Check sheet for the modelled part. Datum: model origin and axes. Units: mm. A direction names the side the tool comes from. Give positions to 0.01 mm unless a question says otherwise; leave off trailing zeros. Order: outer loops, then holes, each group sorted by start corner. A loop starts at its lowest first (then second) coordinate and runs counter-clockwise, first axis right, second up.
```python
from build123d import *

# Parameters (mm, degrees)
ESQUISSE1_W             = 150
ESQUISSE1_H             = 150
BOSS_EXTRU_1_DEPTH      = 5
ESQUISSE2_W             = 12
ESQUISSE2_H             = 60
ESQUISSE2_H_2           = 35
ENL_V_MAT_EXTRU_1_DEPTH = 5


with BuildPart() as part:
    # Esquisse1 → Boss.-Extru.1 (new body)
    with BuildSketch(Plane.XY):
        with Locations((75, 75)):
            Rectangle(ESQUISSE1_W, ESQUISSE1_H)
    extrude(amount=BOSS_EXTRU_1_DEPTH)

    # Esquisse2 → Enlèv. mat.-Extru.1 (cut)
    with BuildSketch(Plane.XY.offset(5)):
        with Locations((26, 90)):
            Rectangle(ESQUISSE2_W, ESQUISSE2_H)
        with Locations((124, 90)):
            Rectangle(ESQUISSE2_W, ESQUISSE2_H)
        with Locations((54, 22.5)):
            Rectangle(ESQUISSE2_W, ESQUISSE2_H_2)
        with Locations((96, 22.5)):
            Rectangle(ESQUISSE2_W, ESQUISSE2_H_2)
    extrude(amount=-ENL_V_MAT_EXTRU_1_DEPTH, mode=Mode.SUBTRACT)


solid = part.part
```
(1) Cross-section at B-B on z = 2.5. Enter the section's corners in (x, y), then the cut area to 3 significant figures.
Response values:
outline: (0, 0) - (150, 0) - (150, 150) - (0, 150) - close; hole (20, 60) - (32, 60) - (32, 120) - (20, 120) - close; hole (48, 5) - (60, 5) - (60, 40) - (48, 40) - close; hole (90, 5) - (102, 5) - (102, 40) - (90, 40) - close; hole (118, 60) - (130, 60) - (130, 120) - (118, 120) - close
area: 20,200 mm2
(2) Cross-section at A-A on y = 87. Enter the section's corners in (x, z).
Response values:
outline: (0, 0) - (20, 0) - (20, 5) - (0, 5) - close; (32, 0) - (118, 0) - (118, 5) - (32, 5) - close; (130, 0) - (150, 0) - (150, 5) - (130, 5) - close
(3) Release check for a two-part mould opening along Y. For faces 1 (the face through (96, 40, 3)), 2 (the face through (74, 150, 2)), 3 (the face through (74, 76, 5)), 4 (the face through (26, 120, 3)) record: released by +Y, released by -Y, zero draft, split by the parting line, or undercut.
Response values:
face 1: undercut
face 2: released by +Y
face 3: zero draft
face 4: undercut
(4) Material ranges on L1, parallel to X at y = 67, z = 2.85; L2, parallel to X at y = 39, z = 2.8; L3, parallel to Y at x = 96, z = 2.45, recorded low to high.
Response values:
L1: x = 0 to 20, 32 to 118, 130 to 150
L2: x = 0 to 48, 60 to 90, 102 to 150
L3: y = 0 to 5, 40 to 150
(5) Set-up check for faces 5 (the face through (74, 0, 2)), 6 (the face through (124, 120, 3)): record each of +Z, -Z, +X, -X, +Y, -Y from which the full face is reachable in a straight line by a thin tool's end or side.
Response values:
face 5: +Z, -Z, +X, -X, -Y
face 6: +Z, -Z
